from build123d import *

# Parameters (mm, degrees)
F0_R      = 6
F1_DEPTH  = 95
F1_FACE_R = 6
F2_DEPTH  = 5
F3_R      = 1
F4_SIZE   = 0.5


with BuildPart() as f1:
    # F0 (on Top) → F1 (new body)
    with BuildSketch(Plane.XY):
        Circle(F0_R)
    extrude(amount=F1_DEPTH)

    # F0 (on Top) + F1_face (on face) → F2 (join)
    with BuildSketch(Plane.XY):
        Polygon((8.9462464611, 5.2881635996), (-0.1065607861, 10.3917585037), (-9.0528072472, 5.103594904), (-8.9462464611, -5.2881635996), (0.1065607861, -10.3917585037), (9.0528072472, -5.103594904), align=None)
        Circle(F0_R, mode=Mode.SUBTRACT)
    with BuildSketch(Plane(origin=(0, 0, 0), x_dir=(1, 0, 0), z_dir=(0, 0, -1))):
        Circle(F1_FACE_R)
    extrude(amount=-F2_DEPTH, dir=(0, 0, 1))

    # F3
    f3_edges = [f1.edges().sort_by_distance(p)[0] for p in [
        (-6, 0, 95),
    ]]
    fillet(f3_edges, radius=F3_R)

    # F4
    f4_edges = [f1.edges().sort_by_distance(p)[0] for p in [
        (4.419843, 7.839961, -5),
        (-4.579684, 7.747677, -5),
        (-8.999527, -0.092284, -5),
        (-4.419843, -7.839961, -5),
        (4.579684, -7.747677, -5),
        (8.999527, 0.092284, -5),
        (-4.579684, 7.747677, 0),
        (-8.999527, -0.092284, 0),
        (-4.419843, -7.839961, 0),
        (4.579684, -7.747677, 0),
        (4.419843, 7.839961, 0),
        (8.999527, 0.092284, 0),
    ]]
    chamfer(f4_edges, length=F4_SIZE)


solid = f1.part
The model under review builds one solid part; all positions refer to its coordinate system, in mm. A direction names the side the tool comes from. Round coordinates to 2 decimals unless told otherwise and drop trailing zeros. Order: outer loops, then holes, each group sorted by start corner. A loop starts at its lowest first (then second) coordinate and runs counter-clockwise, first axis right, second up. Notation, with made-up numbers: (3.25, -15) - (51.25, -15) arc R17 ccw to (51.25, 0) - close; hole circle Ø3 at (56, -15.75). An arc over 180 degrees is marked (long way). Use one line per item in the form item = value.
Q1. Add section A-A on z = 33.5. Give the boundary of the cut face in (x, y), then the cut area to 3 significant figures.
Response values:
outline = circle Ø12 at (0, 0)
area = 113 mm^2
Q2. Clearance check with flat-ended pins moving along their axes: P1, Ø1.5, axis at x = 5, y = 8, coming from the -Z side; P2, Ø6, axis at x = 6, y = -6, coming from the +Z side; P3, Ø4, axis at x = 1, z = 50.5, coming from the +Y side. State where each tip first meets the part, or that it passes through.
Response values:
P1 = -4.83
P2 = 94.87
P3 = 6
Q3. Tool access review of faces 1 (the flat face through (4.359, 7.583, -4.754)), 2 (the flat face through (-6, -2, 0)): name each direction out of +Z, -Z, +X, -X, +Y, -Y from which nothing blocks a thin tool from reaching the whole face with its end or side.
Response values:
face_1 = -Z, +X, +Y
face_2 = +Z
Q4. Add section B-B on y = 0. Give the boundary of the cut face in (x, z), then the cut area to 3 significant figures.
Response values:
outline = (-9, -4.5) - (-8.5, -5) - (8.5, -5) - (9, -4.5) - (9, -0.5) - (8.5, 0) - (6, 0) - (6, 94) arc R1 ccw to (5, 95) - (-5, 95) arc R1 ccw to (-6, 94) - (-6, 0) - (-8.5, 0) - (-9, -0.5) - close
area = 1,230 mm^2
Q5. To check wall thickness, follow line 1 (Z direction, x = 5, y = 5.5); line 2 (Y direction, x = 0.5, z = 47); line 3 (X direction, y = 0.25, z = 7). State the ranges of each line that lie inside material, in increasing order.
Response values:
line_1 = -5 to 0
line_2 = -5.98 to 5.98
line_3 = -5.99 to 5.99
